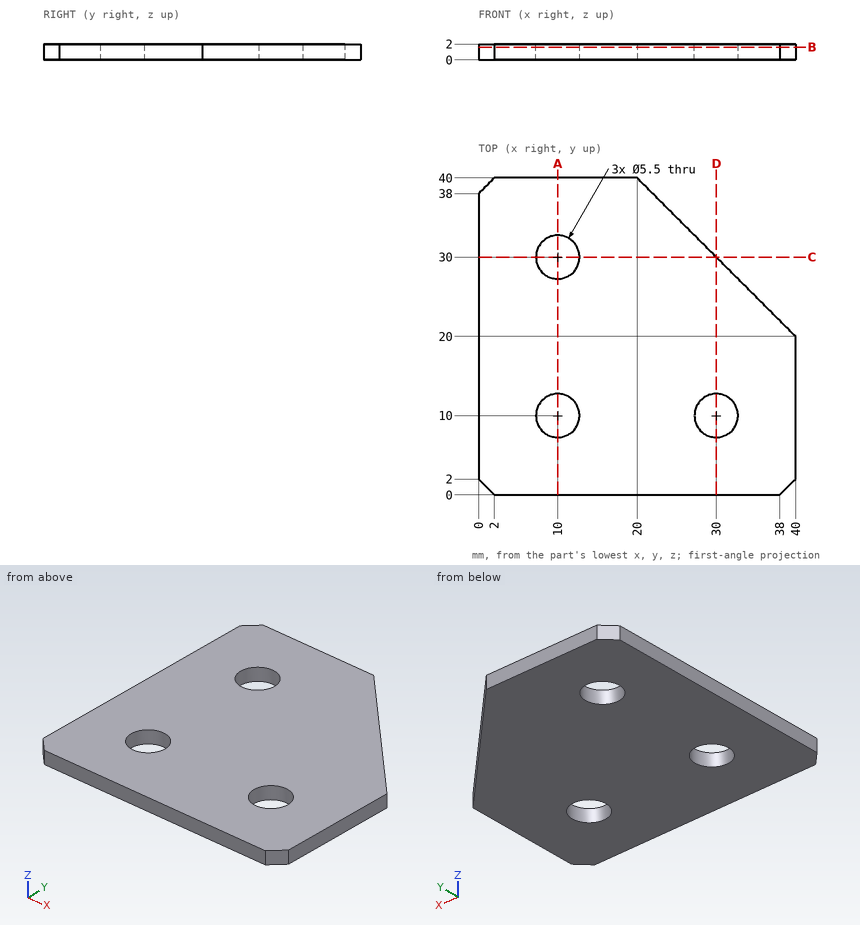
Answer from the drawing. Dimensions are ordinates in mm from the lowest x, y and z of the part. Coordinates: 2 decimals unless noted, no trailing zeros. Loops run counter-clockwise (first coordinate to the right, second up) from the corner with the lowest first, then second, coordinate; pieces in that order, holes last.
1) Section C-C (y = 30) is taken. Give the vertices of the cut face in (x, z), plus the area to 3 significant figures.
Results:
outline: (0, 0) - (7.25, 0) - (7.25, 2) - (0, 2) - close; (12.75, 0) - (30, 0) - (30, 2) - (12.75, 2) - close
area: 49.0 mm2
2) Section A-A (x = 10) is taken. Give the vertices of the cut face in (y, z), plus the area to 3 significant figures.
Results:
outline: (0, 0) - (7.25, 0) - (7.25, 2) - (0, 2) - close; (12.75, 0) - (27.25, 0) - (27.25, 2) - (12.75, 2) - close; (32.75, 0) - (40, 0) - (40, 2) - (32.75, 2) - close
area: 58.0 mm2
3) Flat-ended cylindrical pins translate along their axes: pin 1 (1.5 mm diameter, centred on x = 20, y = 25.5, fed in from -Z); pin 2 (4.5 mm diameter, centred on x = 10, y = 10, fed in from +Z). Find the tip coordinate at first contact, or state that the pin passes through.
Results:
pin 1: stops at z = 0
pin 2: passes through
4) Section B-B (z = 1.6) is taken. Give the vertices of the cut face in (x, y).
Results:
outline: (0, 2) - (2, 0) - (38, 0) - (40, 2) - (40, 20) - (20, 40) - (2, 40) - (0, 38) - close; hole circle Ø5.5 at (10, 10); hole circle Ø5.5 at (10, 30); hole circle Ø5.5 at (30, 10)
5) Consider probe 1 along Y at (x, z) = (10, 1.1); probe 2 along Y at (x, z) = (9, 1.6). Determine where each line is inside the solid, lowest interval first.
Results:
probe 1: y = 0 to 7.25, 12.75 to 27.25, 32.75 to 40
probe 2: y = 0 to 7.44, 12.56 to 27.44, 32.56 to 40
